Study the drawing (mm; zero at the part's minimum x, y, z) and answer. A direction names the side the tool comes from. Coordinates: 2 decimals unless noted, no trailing zeros. Loops run counter-clockwise (first coordinate to the right, second up) from the corner with the lowest first, then second, coordinate; pieces in that order, holes last. Notation, with made-up numbers: (-18, -11) - (9, -11) arc R32 ccw to (9, 17) - close; hole circle Ø10 at (47, 58). An arc over 180 degrees is marked (long way). Write each question's results on one line, items separated by ' | '. Start each with the question number.
(1) Consider line 1 (Z direction, x = 100, y = 24); line 2 (X direction, y = 24, z = 47); line 3 (Y direction, x = 145.5, z = 82). Determine where each line is inside the solid, lowest interval first. Write a range as from..to.
(2) For the marked faces 4 and 5, determine the directions among +Z, -Z, +X, -X, +Y, -Y from which every point of the face is accessible in a straight line to the end or side of a thin tool.
(3) Find section D-D on y = 52.5. Determine the outline of the cut face in (x, z).
(4) Find section C-C on z = 85. Determine the outline of the cut face in (x, y), then the cut area to 3 significant figures.
(5) Find section A-A on y = 37. Determine the outline of the cut face in (x, z).
(6) Determine the mould class of the marked faces 1, 2 and 3 for opening direction X: released by +X, released by -X, zero draft, split by the parting line, or undercut.
(7) Find section B-B on x = 116.5. Determine the outline of the cut face in (y, z).
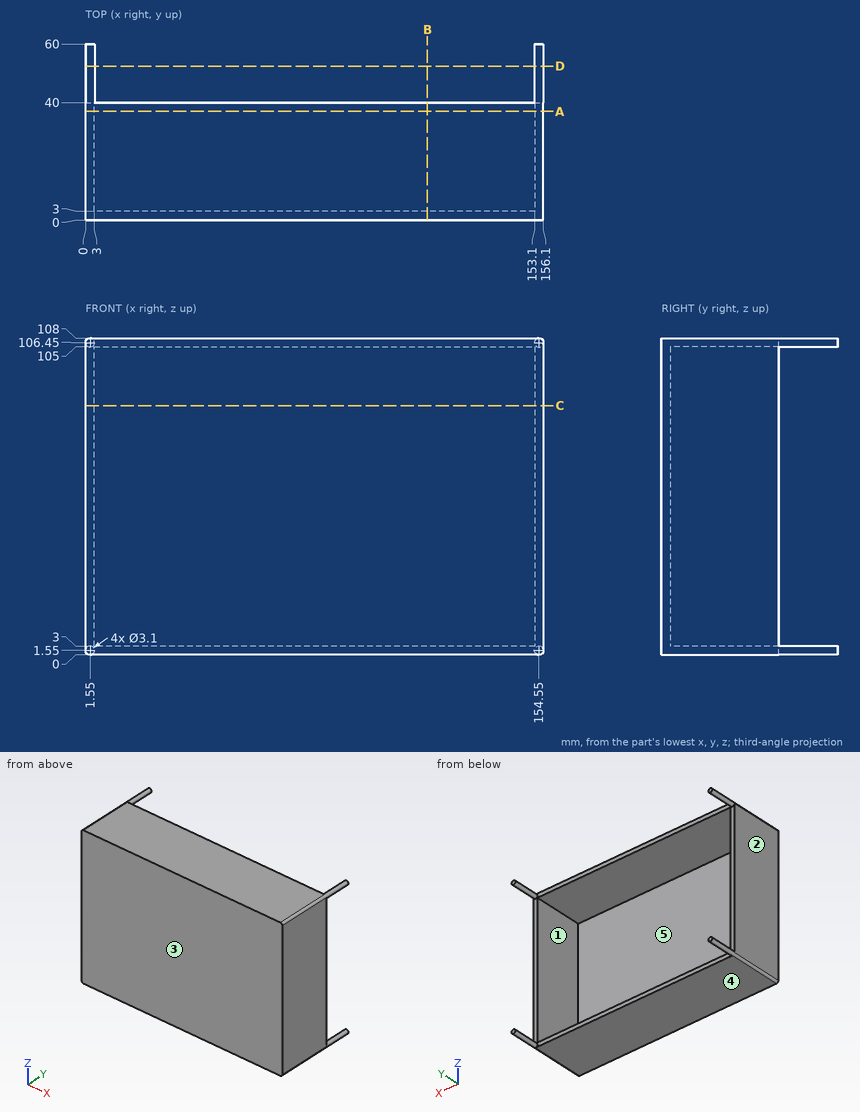
Values:
1) line 1: z = 0..3, 105..108 | line 2: x = 0..3, 153.1..156.1 | line 3: y = 0..3
2) face 4: -Z, +X, -X, +Y, -Y | face 5: +Y
3) outline: circle Ø3.1 at (1.55, 1.55); circle Ø3.1 at (1.55, 106.45); circle Ø3.1 at (154.55, 1.55); circle Ø3.1 at (154.55, 106.45)
4) outline: (0, 0) - (156.1, 0) - (156.1, 40) - (153.1, 40) - (153.1, 3) - (3, 3) - (3, 40) - (0, 40) - close | area: 690 mm²
5) outline: (0, 1.55) arc R1.55 ccw to (1.55, 0) - (154.55, 0) arc R1.55 ccw to (156.1, 1.55) - (156.1, 106.45) arc R1.55 ccw to (154.55, 108) - (1.55, 108) arc R1.55 ccw to (0, 106.45) - close; hole (3, 3) - (153.1, 3) - (153.1, 105) - (3, 105) - close
6) face 1: undercut | face 2: released by -X | face 3: zero draft
7) outline: (0, 0) - (40, 0) - (40, 3) - (3, 3) - (3, 105) - (40, 105) - (40, 108) - (0, 108) - close
